Autodesk Fusion 360 part; units mm, degrees
sketch "Esquisse1" plane through (0, 0, 0) normal (0, 0, 1) x (1, 0, 0)
  circle A0 centre (0, 0) radius 4.5
  circle A1 centre (0, 0) radius 2.9
  circle A2 centre (0, 0) radius 1.7
  dimension "d1" = 5.8
  dimension "d2" = 3.4
  dimension "d3" = 9
extrude "Extrusion1" add sketch "Esquisse1" along normal blind 9 contours A1
extrude "Extrusion2" add sketch "Esquisse1" against normal blind 2 contours A0 | A1 | A2
chamfer "Chanfrein1" distance 1 angle 45 1 edges at (-1.585, 0.6147, 0)
chamfer "Chanfrein2" distance 1.5 angle 45 1 edges at (-4.1955, 1.6273, -2)
chamfer "Chanfrein3" distance 0.7 angle 45 1 edges at (-1.585, 0.6147, 9)
chamfer "Chanfrein4" distance 0.1 angle 45 1 edges at (-2.7037, -1.0487, 9)
chamfer "Chanfrein5" distance 0.1 angle 45 1 edges at (-4.1955, -1.6273, 0)
chamfer "Chanfrein6" distance 0.2 angle 45 1 edges at (-2.7037, -1.0487, 0)
Read the model definition and answer for the solid it produces. Units are mm, in the model's axes. A direction names the side the tool comes from. Coordinates: 2 decimals unless noted, no trailing zeros. Write each loop counter-clockwise with the first axis right and the second up, starting at its lowest first coordinate (ties: lowest second). Pieces come first, ordered by that corner, then holes. Notation, with made-up numbers: (85, 48.25) - (89, 48.25) arc R29 ccw to (89, 78.25) - close; hole circle Ø5 at (19, 75). An arc over 180 degrees is marked (long way). One line per question, with ' | ' between items.
Q1. Find section C-C, the plane z = 3.75. Write down the section's boundary in (x, y), plus the area to 3 significant figures.
Result set:
outline: circle Ø5.8 at (0, 0); hole circle Ø3.4 at (0, 0) | area: 17.3 mm^2
Q2. Find section D-D, the plane z = -1. Write down the section's boundary in (x, y).
Result set:
outline: circle Ø8 at (0, 0)
Q3. Each of these flat-tipped pins is pushed along its axis until it touches: P1, Ø1.5, axis at y = -0.5, z = -1, coming from the -X side; P2, Ø1.1, axis at x = -0.5, y = 0, coming from the +Z side; P3, Ø3, axis at x = 2, z = 3.5, coming from the -Y side. Where does it stop, or does it pass through?
Result set:
P1: x = -4.5 | P2: z = 0.35 | P3: y = -2.86
Q4. For faces 1 (the flat face through (0, 0, -2)), 2 (the flat face through (0, 0, 0)), determine the directions among +Z, -Z, +X, -X, +Y, -Y from which every point of the face is accessible in a straight line to the end or side of a thin tool.
Result set:
face 1: -Z, +X, -X, +Y, -Y | face 2: +Z
Q5. Consider L1, parallel to Y at x = 0, z = 7; L2, parallel to X at y = 1, z = 3.75; L3, parallel to X at y = 1.5, z = 5.75. Determine where each line is inside the solid, lowest interval first. Write a range as [from, to].
Result set:
L1: [-2.9, -1.7], [1.7, 2.9] | L2: [-2.72, -1.37], [1.37, 2.72] | L3: [-2.48, -0.8], [0.8, 2.48]
Q6. Find section A-A, the plane y = 0. Write down the section's boundary in (x, z).
Result set:
outline: (-4.5, -0.5) - (-3, -2) - (3, -2) - (4.5, -0.5) - (4.5, -0.1) - (4.4, 0) - (3.1, 0) - (2.9, 0.2) - (2.9, 8.9) - (2.8, 9) - (2.4, 9) - (1.7, 8.3) - (1.7, 1) - (0.7, 0) - (-0.7, 0) - (-1.7, 1) - (-1.7, 8.3) - (-2.4, 9) - (-2.8, 9) - (-2.9, 8.9) - (-2.9, 0.2) - (-3.1, 0) - (-4.4, 0) - (-4.5, -0.1) - close
